Geometry: final body of the model. Coordinates: model frame, mm. Face numbers are marked on the shaded views. Give positions to 0.01 mm unless a question says otherwise; leave off trailing zeros. Write each loop counter-clockwise with the first axis right and the second up, starting at its lowest first coordinate (ties: lowest second). Pieces come first, ordered by that corner, then holes. Notation, with made-up numbers: (85, -10.75) -> (126, -10.75) arc R14 cw to (126, 5.25) -> close; hole circle Ø11 at (79, 48.25). An arc over 180 degrees is marked (long way). Answer in a Markdown table with one row per item. Add a question column.
Item 1: Section query B-B on x = 22. Output: boundary loops of the cut face in (y, z), plus the area to 3 significant figures.
Item 2: Draft query along Y for the marked faces 1, 2 and 3. Return one class per face: +Y half, -Y half, draft (parallel to the pull), parting line (faces both ways), or undercut.
Item 3: Section query D-D on z = 0.7. Output: boundary loops of the cut face in (x, y), plus the area to 3 significant figures.
Item 4: Section query A-A on y = 12.75. Output: boundary loops of the cut face in (x, z).
Item 5: Material intervals for probe 1 along X at (y, z) = (15, 4.05); probe 2 along Y at (x, z) = (6, 1.2); probe 3 along Z at (x, y) = (16.25, 19), sorted ascending. Write a range as from..to.
Item 6: Section query C-C on y = 14. Output: boundary loops of the cut face in (x, z).
Item 7: First-contact query: P1, Ø2, axis at y = 18.5, z = 0.5, coming from the +X side; P2, Ø1.5, axis at x = 9, y = 17, coming from the +Z side. Flat tips, straight axial feed; report the tip coordinate or a pass-through.
```python
from build123d import *

# Parameters (mm, degrees)
SKETCH_1_R      = 5
SKETCH_1_R_2    = 2.817909336
EXTRUDE_1_DEPTH = 5
SKETCH_2_R      = 0.976753742
EXTRUDE_2_DEPTH = 2


with BuildPart() as part:
    # 草图1 → 凸台-拉伸1 (new body)
    with BuildSketch(Plane.XY):
        with Locations((20.979563361, 15.154638973)):
            Circle(SKETCH_1_R)
        with Locations((20.979563361, 15.154638973)):
            Circle(SKETCH_1_R_2, mode=Mode.SUBTRACT)
    extrude(amount=EXTRUDE_1_DEPTH)

    # 草图2 → 凸台-拉伸2 (add)
    with BuildSketch(Plane(origin=(0, 0, 0), x_dir=(-1, 0, 0), z_dir=(0, 0, -1))):
        with BuildLine():
            Line((-20.979563361, 20.154638973), (-5.979563361, 17.717173943))
            ThreePointArc((-5.979563361, 17.717173943), (-3.819583674, 15.557194255), (-5.979563361, 13.397214568))
            Line((-5.979563361, 13.397214568), (-20.979563361, 10.154638973))
            Line((-20.979563361, 10.154638973), (-20.873226182, 11.0026068))
            Line((-20.873226182, 11.0026068), (-17.89105269, 13.59821912))
            Line((-17.89105269, 13.59821912), (-17.479167483, 16.13293368))
            Line((-17.479167483, 16.13293368), (-20.979563361, 20.154638973))
        make_face()
        with Locations((-5.979563361, 15.557194255)):
            Circle(SKETCH_2_R, mode=Mode.SUBTRACT)
    extrude(amount=-EXTRUDE_2_DEPTH)


solid = part.part
```
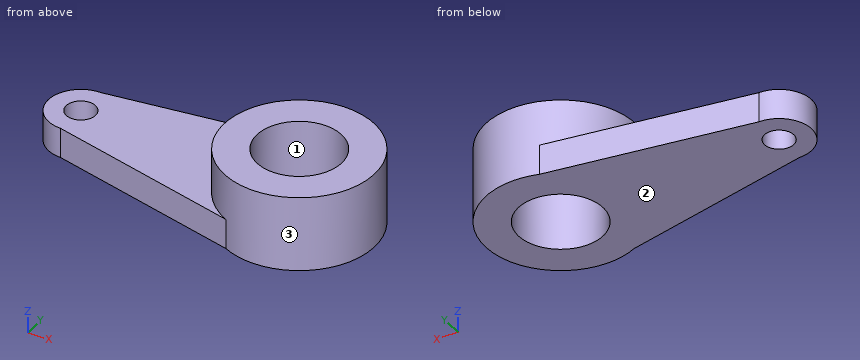
Findings below:
| question | item | result |
|---|---|---|
| 1 | outline | (10.26, 0) -> (12.53, 0) -> (12.53, 5) -> (10.26, 5) -> close; (17.78, 0) -> (20.05, 0) -> (20.05, 5) -> (17.78, 5) -> close |
| 1 | area | 22.7 mm^2 |
| 2 | face 1 | undercut |
| 2 | face 2 | draft |
| 2 | face 3 | parting line |
| 3 | outline | (5.98, 13.4) -> (18.91, 10.6) arc R5 ccw (long way) to (19.4, 19.9) -> (5.98, 17.72) arc R2.16 ccw to start; hole circle Ø1.95 at (5.98, 15.56); hole circle Ø5.64 at (20.98, 15.15) |
| 3 | area | 126 mm^2 |
| 4 | outline | (8.97, 0) -> (19.51, 0) -> (19.51, 5) -> (16.6, 5) -> (16.6, 2) -> (8.97, 2) -> close; (22.45, 0) -> (25.36, 0) -> (25.36, 5) -> (22.45, 5) -> close |
| 5 | probe 1 | x = 15.98..18.17, 23.79..25.98 |
| 5 | probe 2 | y = 13.39..14.58, 16.53..17.72 |
| 5 | probe 3 | z = 0..2 |
| 6 | outline | (4.48, 0) -> (18.41, 0) -> (18.41, 5) -> (16.11, 5) -> (16.11, 2) -> (4.48, 2) -> close; (23.55, 0) -> (25.84, 0) -> (25.84, 5) -> (23.55, 5) -> close |
| 7 | P1 | stops at x = 25.4 |
| 7 | P2 | stops at z = 2 |
